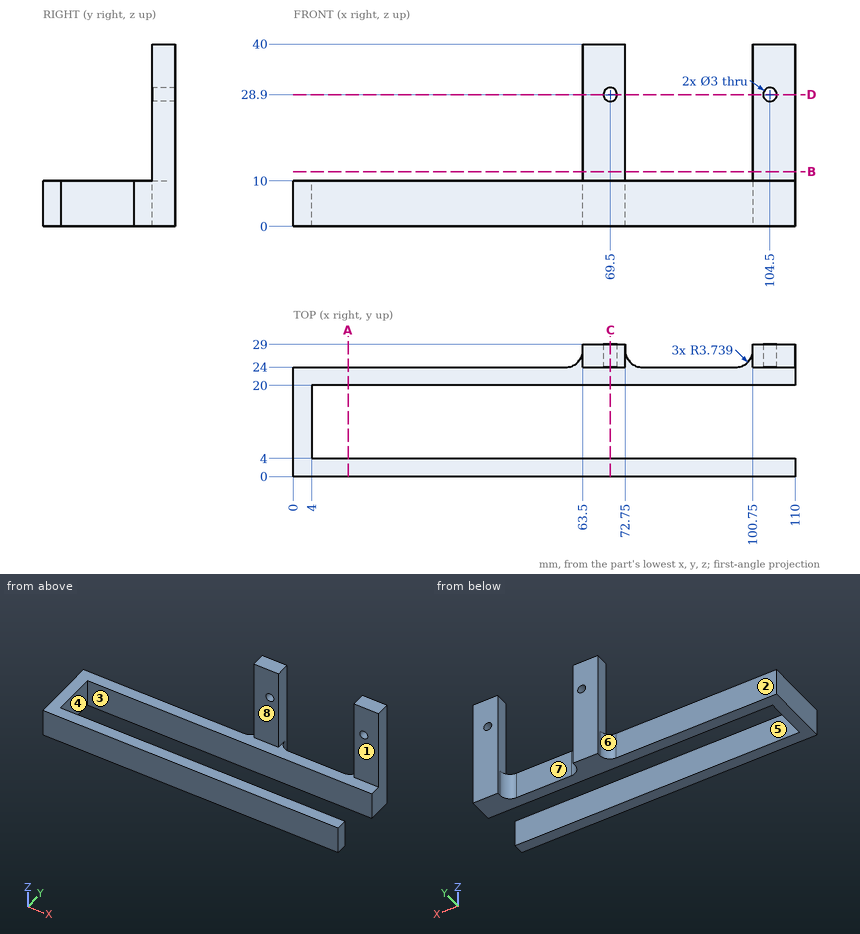
Check sheet for the drawn part. Datum: minimum x, y, z corner. Units: mm. A direction names the side the tool comes from. Round coordinates to 2 decimals unless told otherwise and drop trailing zeros. Loops run counter-clockwise (first coordinate to the right, second up) from the corner with the lowest first, then second, coordinate; pieces in that order, holes last.
Item 1: Mould release check, pull along Y, two halves, no side actions. Record for the marked faces 1, 2, 3 and 4: pulls with the +Y half, pulls with the -Y half, needs draft (parallel to the pull), parting line crosses it, or undercut.
Item 2: Cross-section at A-A on x = 12. Record the boundary of the cut face in (y, z), then the cut area to 3 significant figures.
Item 3: Cross-section at B-B on z = 12. Record the boundary of the cut face in (x, y).
Item 4: Gauge pin test, flat ends, axial feed: pin 1 (11 mm diameter, centred on x = 38.5, z = 4, fed in from +Y); pin 2 (5 mm diameter, centred on y = 11.5, z = 7, fed in from +X); pin 3 (4.5 mm diameter, centred on x = 66.5, z = 17.5, fed in from -Y); pin 4 (1.8 mm diameter, centred on x = 69.5, z = 28.9, fed in from -Y). Record the tip position at first contact, or that the pin passes through.
Item 5: Cross-section at D-D on z = 28.9. Record the boundary of the cut face in (x, y).
Item 6: Cross-section at C-C on x = 69.5. Record the boundary of the cut face in (y, z).
Item 7: Access from +Z, -Z, +X, -X, +Y, -Y to the whole of each face (thin tool, end or side, straight path). Record for the marked faces 5, 6, 7 and 8.
Item 8: Thickness scan on line 1 (Z direction, x = 104.5, y = 25.6); line 2 (Y direction, x = 84.5, z = 3); line 3 (X direction, y = 24.5, z = 27). Record the ranges inside material, lowest first.
Answer sheet:
1. face 1: pulls with the -Y half
1. face 2: pulls with the +Y half
1. face 3: undercut
1. face 4: undercut
2. outline: (0, 0) - (4, 0) - (4, 10) - (0, 10) - close; (20, 0) - (24, 0) - (24, 10) - (20, 10) - close
2. area: 80.0 mm2
3. outline: (63.5, 24) - (72.75, 24) - (72.75, 29) - (63.5, 29) - close; (100.75, 24) - (110, 24) - (110, 29) - (100.75, 29) - close
4. pin 1: stops at y = 24
4. pin 2: stops at x = 4
4. pin 3: stops at y = 24
4. pin 4: passes through
5. outline: (63.5, 24) - (68, 24) - (68, 29) - (63.5, 29) - close; (71, 24) - (72.75, 24) - (72.75, 29) - (71, 29) - close; (100.75, 24) - (103, 24) - (103, 29) - (100.75, 29) - close; (106, 24) - (110, 24) - (110, 29) - (106, 29) - close
6. outline: (0, 0) - (4, 0) - (4, 10) - (0, 10) - close; (20, 0) - (29, 0) - (29, 27.4) - (24, 27.4) - (24, 10) - (20, 10) - close; (24, 30.4) - (29, 30.4) - (29, 40) - (24, 40) - close
7. face 5: +Z, -Z, +X
7. face 6: +Z, -Z, -X, +Y
7. face 7: +Z, -Z, +Y
7. face 8: +Z, +X, -X, -Y
8. line 1: z = 0 to 27.4, 30.4 to 40
8. line 2: y = 0 to 4, 20 to 24
8. line 3: x = 63.5 to 72.75, 100.75 to 110
